Could you check a few things on this model? Use its own coordinates, in mm. A direction names the side the tool comes from. Give positions to 0.01 mm unless a question says otherwise; leave off trailing zeros. Write each loop counter-clockwise with the first axis right and the second up, starting at its lowest first coordinate (ties: lowest second). Pieces come first, ordered by that corner, then holes. Notation, with made-up numbers: M -13.75,59.5 L -9.75,59.5 A28 cw -9.75,96.5 Z; hole C -11,88.25 d11. An arc over 180 degrees is marked long. Answer as a JSON object with one key per item and string values. Group by question number.
```python
from build123d import *

# Parameters (mm, degrees)
F0_R     = 4.5
F1_DEPTH = 6


with BuildPart() as f1:
    # F0 (on Front) → F1 (new body)
    with BuildSketch(Plane.XZ):
        with BuildLine():
            ThreePointArc((-140.218107, -62.01527), (-128.222675, -63.196717), (-124.723737, -51.662263))
            ThreePointArc((-124.723737, -51.662263), (-135, 0), (-124.723737, 51.662263))
            ThreePointArc((-124.723737, 51.662263), (-127.993204, 63.038471), (-139.812549, 62.3977))
            Line((-139.812549, 62.3977), (-210, 0))
            Line((-210, 0), (-210, -35))
            Line((-210, -35), (-170.547086, -35))
            ThreePointArc((-170.547086, -35), (-167.485618, -35.608964), (-164.890232, -37.343146))
            Line((-164.890232, -37.343146), (-140.218107, -62.01527))
        make_face()
        with Locations((-133.500592, -55.297756)):
            Circle(F0_R, mode=Mode.SUBTRACT)
        with Locations((-133.500592, 55.297756)):
            Circle(F0_R, mode=Mode.SUBTRACT)
    extrude(amount=F1_DEPTH)


solid = f1.part
```
1) We'd pull the mould along X, two halves only. Please class faces 1 (the cylindrical face through (-137.996, -2.958, 55.496)), 2 (the cylindrical face through (-137.996, -2.958, -55.1)), 3 (the flat face through (-174.41, -2.96, 31.64)), 4 (the cylindrical face through (-135, -3, -0.7)): released by +X, released by -X, zero draft, split by the parting line, or undercut.
2) I'm going to push flat-ended pins straight in: pin 1 (3 mm diameter, centred on x = -184, y = -1, fed in from -Z); pin 2 (1.5 mm diameter, centred on y = -1, z = 24.5, fed in from -X); pin 3 (3 mm diameter, centred on x = -162.5, y = -5, fed in from -Z). Where does each tip first touch, or does it pass through?
3) Please list where these lines run through material, in increasing order: line 1 along X through (y, z) = (-4.4, -1.5); line 2 along X through (y, z) = (-3.1, -58); line 3 along X through (y, z) = (-1.8, 55). Write a range as from..to.
4) If we section it at A-A, the plane y = -2.95: List the corners of the cut face in (x, z) for me.
5) For faces 5 (the flat face through (-191, -3, -35)), 6 (the flat face through (-158, -6, 1)), which set-ups out of +Z, -Z, +X, -X, +Y, -Y let a thin tool reach every point of the face, with its end or its side?
6) If we section it at B-B, the plane x = -173: List the corners of the cut face in (y, z) for me.
7) If we section it at C-C, the plane z = -15: List the corners of the cut face in (x, y) for me.
Taken from the geometry:
{
 "1": {"face 1": "undercut", "face 2": "undercut", "face 3": "released by -X", "face 4": "released by +X"},
 "2": {"pin 1": "z = -35", "pin 2": "x = -183.29", "pin 3": "z = -41.23"},
 "3": {"line 1": "-210..-134.99", "line 2": "-144.23..-137.1, -129.9..-124.39", "line 3": "-148.13..-137.99, -129.01..-124.01"},
 "4": {"outline": "M -210,-35 L -170.55,-35 A8 cw -164.89,-37.34 L -140.22,-62.02 A9.5 ccw -124.72,-51.66 A135 cw -124.72,51.66 A9.5 ccw -139.81,62.4 L -210,0 Z; hole C -133.5,-55.3 d9; hole C -133.5,55.3 d9"},
 "5": {"face 5": "-Z, -X, +Y, -Y", "face 6": "+Z, -Z, +X, -X, -Y"},
 "6": {"outline": "M -6,-35 L 0,-35 L 0,32.89 L -6,32.89 Z"},
 "7": {"outline": "M -210,-6 L -134.16,-6 L -134.16,0 L -210,0 Z"}
}
